Answer from the drawing. Dimensions are ordinates in mm from the lowest x, y and z of the part. A direction names the side the tool comes from. Give positions to 0.01 mm unless a question says otherwise; leave off trailing zeros. Loops run counter-clockwise (first coordinate to the right, second up) from the corner with the lowest first, then second, coordinate; pieces in that order, holes last. Notation, with made-up numbers: (83.25, 24) - (91.25, 24) arc R21 cw to (91.25, 56) - close; hole circle Ø2 at (58, 62). An arc over 180 degrees is marked (long way). One line per item, written item: value.
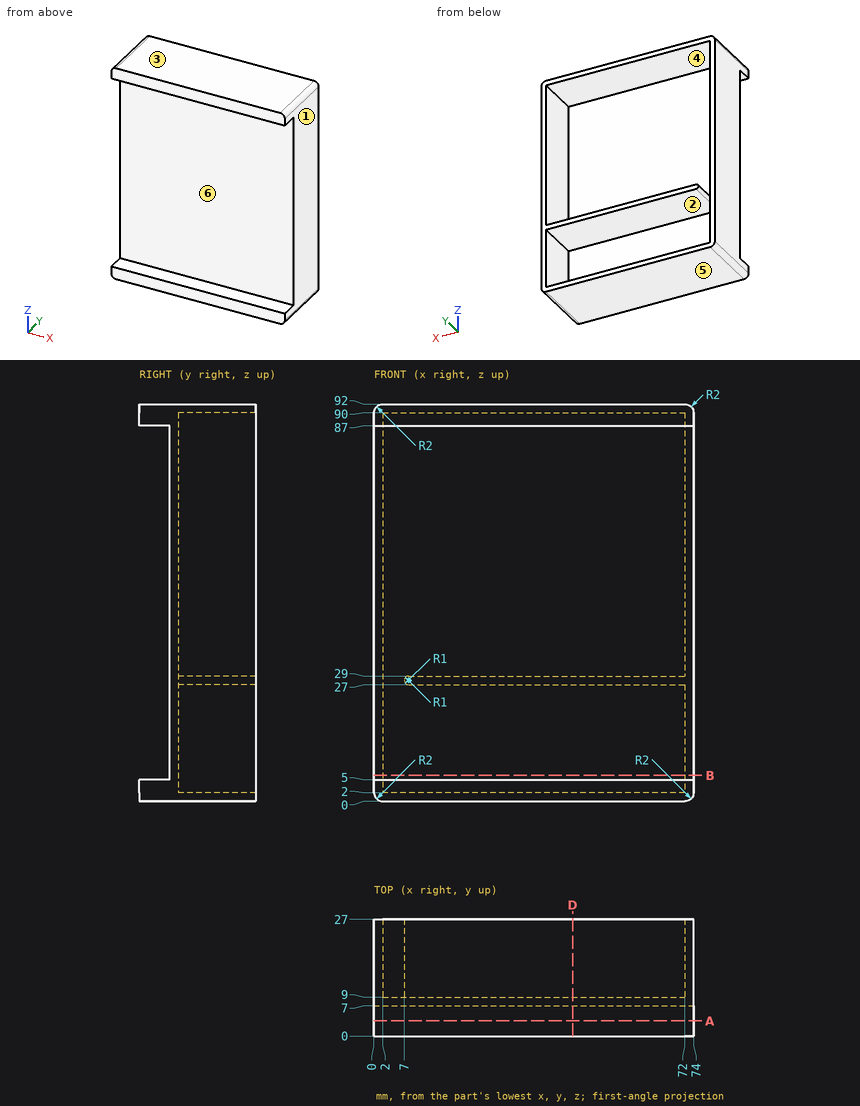
1. A flat-ended cylindrical pin translates along its axis: pin 1 Ø8 at (x, z) = (49.5, 39) entering from -Y. Find the tip coordinate at first contact, or state that the pin passes through.
Output:
pin 1: stops at y = 7
2. Find the intervals of material crossed by line 1 along Z through (x, y) = (29, 22.5); line 2 along Z through (x, y) = (38, 2.5); line 3 along X through (y, z) = (12.5, 11), in increasing order.
Output:
line 1: z = 0 to 2, 27 to 29, 90 to 92
line 2: z = 0 to 5, 87 to 92
line 3: x = 0 to 2, 72 to 74
3. Section D-D (x = 46) is taken. Write down the section's boundary in (y, z).
Output:
outline: (0, 0) - (27, 0) - (27, 2) - (9, 2) - (9, 27) - (27, 27) - (27, 29) - (9, 29) - (9, 90) - (27, 90) - (27, 92) - (0, 92) - (0, 87) - (7, 87) - (7, 5) - (0, 5) - close
4. The mould has two halves that part along Z. Classify the marked faces 1, 2 and 3: released by +Z, released by -Z, zero draft, split by the parting line, or undercut.
Output:
face 1: zero draft
face 2: undercut
face 3: released by +Z
5. Section A-A (y = 3.5) is taken. Write down the section's boundary in (x, z).
Output:
outline: (0, 2) arc R2 ccw to (2, 0) - (72, 0) arc R2 ccw to (74, 2) - (74, 5) - (0, 5) - close; (0, 87) - (74, 87) - (74, 90) arc R2 ccw to (72, 92) - (2, 92) arc R2 ccw to (0, 90) - close
6. Section B-B (z = 6) is taken. Write down the section's boundary in (x, y).
Output:
outline: (0, 7) - (74, 7) - (74, 27) - (72, 27) - (72, 9) - (2, 9) - (2, 27) - (0, 27) - close
7. For the marked faces 4, 5 and 6, determine the directions among +Z, -Z, +X, -X, +Y, -Y from which every point of the face is accessible in a straight line to the end or side of a thin tool.
Output:
face 4: +Y
face 5: -Z, +X, -X, +Y, -Y
face 6: +X, -X, -Y
